Read the model definition and answer for the solid it produces. Units are mm, in the model's axes. Face numbers are marked on the shaded views. A direction names the side the tool comes from. Coordinates: 2 decimals unless noted, no trailing zeros. Order: outer loops, then holes, each group sorted by start corner. A loop starts at its lowest first (then second) coordinate and runs counter-clockwise, first axis right, second up.
```python
from build123d import *

# Parameters (mm, degrees)
SKETCH_1_W          = 61
SKETCH_1_H          = 33.5
EXTRUDE_1_DEPTH     = 50
SKETCH_2_W          = 55
SKETCH_2_H          = 44
CUT_EXTRUDE_1_DEPTH = 30.5
FILLET_3_R          = 27.5
FILLET_4_R          = 30.5
SKETCH_3_R          = 23.5
CUT_EXTRUDE_2_DEPTH = 30.5
SKETCH_5_R          = 16
CUT_EXTRUDE_4_DEPTH = 30.5
FILLET_5_R          = 4
FILLET_6_R          = 2
SKETCH_6_W          = 61
SKETCH_6_H          = 3
CUT_EXTRUDE_5_DEPTH = 400


with BuildPart() as part:
    # 스케치1 → 보스-돌출1 (new body)
    with BuildSketch(Plane(origin=(0, 0, 0), x_dir=(1, 0, 0), z_dir=(0, 1, 0))):
        Rectangle(SKETCH_1_W, SKETCH_1_H)
    extrude(amount=EXTRUDE_1_DEPTH)

    # 스케치2 → 컷-돌출1 (cut)
    with BuildSketch(Plane(origin=(0, 0, -16.75), x_dir=(-1, 0, 0), z_dir=(0, 0, -1))):
        with Locations((0, 25)):
            Rectangle(SKETCH_2_W, SKETCH_2_H)
    extrude(amount=-CUT_EXTRUDE_1_DEPTH, mode=Mode.SUBTRACT)

    # 필렛3
    fillet_3_edges = [part.edges().sort_by_distance(p)[0] for p in [
        (-27.5, 25, 13.75),
        (27.5, 25, 13.75),
    ]]
    fillet(fillet_3_edges, radius=FILLET_3_R - 0.0001)  # a hair under: the kernel refuses the full size

    # 필렛4
    fillet_4_edges = [part.edges().sort_by_distance(p)[0] for p in [
        (-30.5, 25, 16.75),
        (30.5, 25, 16.75),
    ]]
    fillet(fillet_4_edges, radius=FILLET_4_R - 0.0001)  # a hair under: the kernel refuses the full size

    # 스케치3 → 컷-돌출2 (cut)
    with BuildSketch(Plane.XZ):
        with Locations((0, -13.75)):
            Circle(SKETCH_3_R)
    extrude(amount=-CUT_EXTRUDE_2_DEPTH, mode=Mode.SUBTRACT)

    # 스케치5 → 컷-돌출4 (cut)
    with BuildSketch(Plane.XZ.offset(-47)):
        with Locations((0, -13.75)):
            Circle(SKETCH_5_R)
    extrude(amount=-CUT_EXTRUDE_4_DEPTH, mode=Mode.SUBTRACT)

    # 필렛5
    fillet_5_edges = [part.edges().sort_by_distance(p)[0] for p in [
        (-15.716233646, 48.5, -16.75),
        (15.716233646, 48.5, -16.75),
    ]]
    fillet(fillet_5_edges, radius=FILLET_5_R)

    # 필렛6
    fillet_6_edges = [part.edges().sort_by_distance(p)[0] for p in [
        (-23.307724042, 1.5, -16.75),
        (23.307724042, 1.5, -16.75),
    ]]
    fillet(fillet_6_edges, radius=FILLET_6_R)

    # 스케치6 → 컷-돌출5 (cut)
    with BuildSketch(Plane(origin=(0, 0, -16.75), x_dir=(-1, 0, 0), z_dir=(0, 0, -1))):
        with Locations((0, 48.5)):
            Rectangle(SKETCH_6_W, SKETCH_6_H)
    extrude(amount=-CUT_EXTRUDE_5_DEPTH, mode=Mode.SUBTRACT)


solid = part.part
```
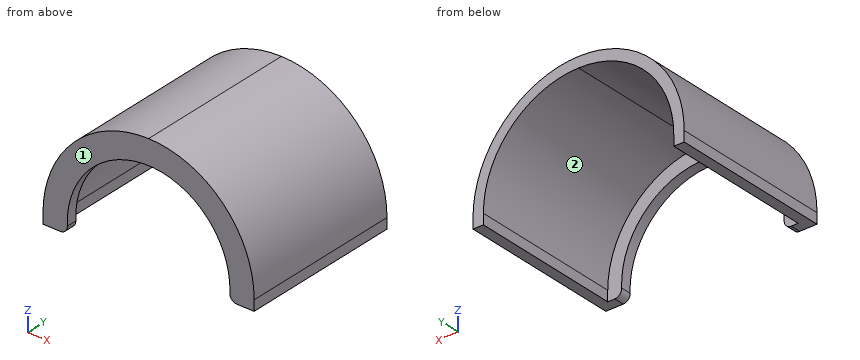
1) Which of the six approach directions +Z, -Z, +X, -X, +Y, -Y give full straight-line access (tool end or side, diameter ignored) to the marked faces 1 and 2?
A:
face 1: +Z, -Z, +X, -X, -Y
face 2: -Z, +Y
2) Straight lines are drawn through the part: line 1 (X direction, y = 37, z = -14); line 2 (X direction, y = 26.5, z = 6); line 3 (Y direction, x = 14, z = 8). For each, find the intervals that lie inside material, in ascending order.
A:
line 1: x = -30.5 to -27.5, 27.5 to 30.5
line 2: x = -23.24 to -19.14, 19.14 to 23.24
line 3: y = 0 to 3
3) A cutting plane is placed at A-A, the plane z = 9. Determine the outline of the cut face in (x, y).
A:
outline: (-20.31, 0) - (-5.89, 0) - (-5.89, 3) - (-15.45, 3) - (-15.45, 47) - (-20.31, 47) - close; (5.89, 0) - (20.31, 0) - (20.31, 47) - (15.45, 47) - (15.45, 3) - (5.89, 3) - close
4) A cutting plane is placed at C-C, the plane x = 8. Determine the outline of the cut face in (y, z), and give its area (3 significant figures).
A:
outline: (0, 8.35) - (3, 8.35) - (3, 12.56) - (47, 12.56) - (47, 15.68) - (0, 15.68) - close
area: 159 mm2
5) A cutting plane is placed at D-D, the plane z = -6.5. Determine the outline of the cut face in (x, y).
A:
outline: (-29.63, 0) - (-22.35, 0) - (-22.35, 3) - (-26.53, 3) - (-26.53, 47) - (-29.63, 47) - close; (22.35, 0) - (29.63, 0) - (29.63, 47) - (26.53, 47) - (26.53, 3) - (22.35, 3) - close
6) Flat-ended cylindrical pins translate along their axes: pin 1 Ø3 at (y, z) = (27, 13) entering from +X; pin 2 Ø2 at (x, y) = (-11.5, 39.5) entering from -Z; pin 3 Ø2 at (y, z) = (19.5, 4.5) entering from -X. Find the tip coordinate at first contact, or state that the pin passes through.
A:
pin 1: stops at x = 17.11
pin 2: stops at z = 10.74
pin 3: stops at x = -25.15
